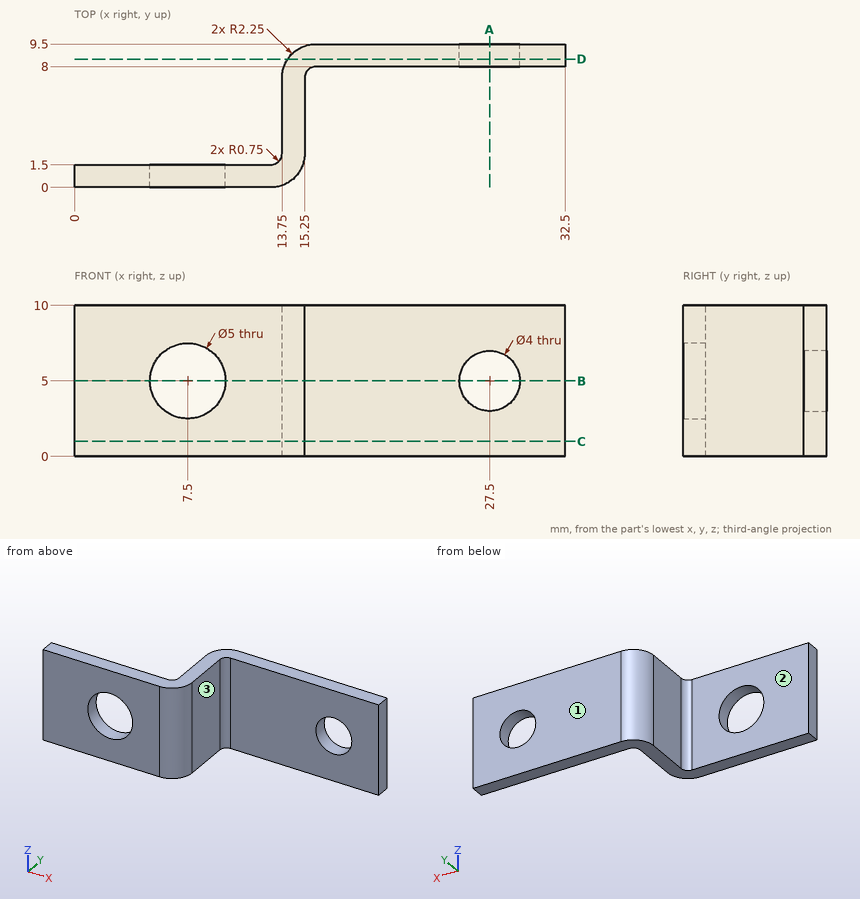
Study the drawing (mm; zero at the part's minimum x, y, z) and answer. A direction names the side the tool comes from. Give positions to 0.01 mm unless a question says otherwise; leave off trailing zeros. Write each loop counter-clockwise with the first axis right and the second up, starting at its lowest first coordinate (ties: lowest second). Pieces come first, ordered by that corner, then holes.
Item 1: Section B-B, the plane z = 5 is taken. Write down the section's boundary in (x, y), plus the area to 3 significant figures.
Item 2: Find the intervals of material crossed by line 1 along Y through (x, z) = (18, 6); line 2 along Y through (x, z) = (9, 8.5); line 3 along X through (y, z) = (4, 6.75), in increasing order.
Item 3: Section D-D, the plane y = 8.5 is taken. Write down the section's boundary in (x, z).
Item 4: Section A-A, the plane x = 27.5 is taken. Write down the section's boundary in (y, z), plus the area to 3 significant figures.
Item 5: Flat-ended cylindrical pins translate along their axes: P1, Ø3.5, axis at x = 27.5, z = 5, coming from the +Y side; P2, Ø1.5, axis at y = 4.5, z = 5.5, coming from the -X side; P3, Ø6, axis at x = 7.5, z = 5, coming from the -Y side; P4, Ø5, axis at x = 9, z = 6.5, coming from the +Y side. Find the tip coordinate at first contact, or state that the pin passes through.
Item 6: Which of the six approach directions +Z, -Z, +X, -X, +Y, -Y give full straight-line access (tool end or side, diameter ignored) to the marked faces 1, 2 and 3?
Item 7: Section C-C, the plane z = 1 is taken. Write down the section's boundary in (x, y), plus the area to 3 significant figures.
Completed:
1. outline: (0, 0) - (5, 0) - (5, 1.5) - (0, 1.5) - close; (10, 0) - (13, 0) arc R2.25 ccw to (15.25, 2.25) - (15.25, 7.25) arc R0.75 cw to (16, 8) - (25.5, 8) - (25.5, 9.5) - (16, 9.5) arc R2.25 ccw to (13.75, 7.25) - (13.75, 2.25) arc R0.75 cw to (13, 1.5) - (10, 1.5) - close; (29.5, 8) - (32.5, 8) - (32.5, 9.5) - (29.5, 9.5) - close
1. area: 45.3 mm2
2. line 1: y = 8 to 9.5
2. line 2: y = 0 to 1.5
2. line 3: x = 13.75 to 15.25
3. outline: (14.13, 0) - (32.5, 0) - (32.5, 10) - (14.13, 10) - close; hole circle Ø4 at (27.5, 5)
4. outline: (8, 0) - (9.5, 0) - (9.5, 3) - (8, 3) - close; (8, 7) - (9.5, 7) - (9.5, 10) - (8, 10) - close
4. area: 9.00 mm2
5. P1: passes through
5. P2: stops at x = 13.75
5. P3: stops at y = 0
5. P4: stops at y = 1.5
6. face 1: +Z, -Z, +X, -X, +Y
6. face 2: +Z, -Z, -X, +Y
6. face 3: +Z, -Z, +X, -Y
7. outline: (0, 0) - (13, 0) arc R2.25 ccw to (15.25, 2.25) - (15.25, 7.25) arc R0.75 cw to (16, 8) - (32.5, 8) - (32.5, 9.5) - (16, 9.5) arc R2.25 ccw to (13.75, 7.25) - (13.75, 2.25) arc R0.75 cw to (13, 1.5) - (0, 1.5) - close
7. area: 58.8 mm2
